Geometry: final body of the model. Coordinates: model frame, mm. A direction names the side the tool comes from. Give positions to 0.01 mm unless a question says otherwise; leave off trailing zeros. Loops run counter-clockwise (first coordinate to the right, second up) from the corner with the lowest first, then second, coordinate; pieces in that order, holes last. Notation, with made-up numbers: (79.25, 9) -> (99.25, 9) arc R13 cw to (99.25, 26) -> close; hole circle Ø3 at (12, 8.5). An arc over 180 degrees is marked (long way). Answer in a Markdown table with one row per item. Add a question column.
1) Section query B-B (x = -6). Return the cut outline in (y, z) (3 decimals).
2) Section query C-C (z = 23). Return the cut outline in (x, y) (3 decimals).
3) Access query for faces 4 (the cylindrical face through (-8.136, -0.954, 112.816)), 5 (the flat face through (8, 0, 90.998)). Directions: +Z, -Z, +X, -X, +Y, -Y. A direction counts if a zero-diameter tool reaches every point of the face in a straight line with its end or side. Return the directions, or none.
4) First-contact query: P1, Ø2, axis at x = -30.5, y = -1, coming from the -Z side; P2, Ø1.9, axis at x = 7, y = -1.5, coming from the +Z side; P3, Ø1, axis at y = 1.5, z = 59, coming from the -X side. Flat tips, straight axial feed; report the tip coordinate or a pass-through.
5) Section query A-A (y = 0). Return the cut outline in (x, z).
6) Line query: line 1 (Z direction, x = -16, y = 1.75); line 2 (X direction, y = -0.25, z = 57); line 3 (Z direction, x = -1, y = 1). Output: solid intervals per line, ascending. Write a range as from..to.
7) Draft query along X for faces 1 (the flat face through (8, 0, -90.998)), 2 (the cylindrical face through (-8.136, -0.954, -112.816)), 3 (the cylindrical face through (-31.02, -2.15, -98.66)). Return one class per face: +X half, -X half, draft (parallel to the pull), parting line (faces both ways), or undercut.
```python
from build123d import *

# Parameters (mm, degrees)
SKETCH3_R = 3.175


with BuildPart() as part:
    # Sweep1: sweep along a path in Sketch2
    with BuildLine(Plane(origin=(0, 0, 0), x_dir=(1, 0, 0), z_dir=(0, 1, 0))) as sweep1_path:
        Line((-42.005520706, 0), (-42.005520706, 74.510370248))
        ThreePointArc((-42.005520706, 74.510370248), (-41.43579821, 78.271535981), (-39.777746269, 81.695249631))
        Line((-39.777746269, 81.695249631), (-18.645117879, 112.496831598))
        ThreePointArc((-18.645117879, 112.496831598), (-15.912495952, 114.928072333), (-12.361782541, 115.805903968))
        Line((-12.361782541, 115.805903968), (-4.027166859, 115.805903968))
        ThreePointArc((-4.027166859, 115.805903968), (4.766000348, 112.163654854), (8.408249461, 103.370487647))
        Line((8.408249461, 103.370487647), (8.408249461, 90.998440491))
    # Sketch3 → Sweep1 (sweep)
    with BuildSketch(Plane.XY):
        with Locations((-42.04385452, 0)):
            Circle(SKETCH3_R)
    sweep1 = sweep(path=sweep1_path.line)

    # Mirror2: Sweep1 across plane
    add(sweep1.mirror(Plane(origin=(-42.04385452, 0, 0), x_dir=(1, 0, 0), z_dir=(0, 0, 1))))


solid = part.part
```
Evaluation:
| question | item | result |
|---|---|---|
| 1 | outline | circle Ø6.35 at (0, -115.844); circle Ø6.35 at (0, 115.844) |
| 2 | outline | circle Ø6.35 at (-42.044, 0) |
| 3 | face 4 | none |
| 3 | face 5 | +X, +Y, -Y |
| 4 | P1 | z = -102.15 |
| 4 | P2 | z = 115.01 |
| 4 | P3 | x = -45.06 |
| 5 | outline | (-45.22, -74.51) arc R15.91 ccw to (-42.43, -83.51) -> (-21.29, -114.31) arc R10.83 ccw to (-12.36, -119.02) -> (-4.03, -119.02) arc R15.65 ccw to (11.62, -103.37) -> (11.62, -91) -> (5.27, -91) -> (5.27, -103.37) arc R9.3 cw to (-4.03, -112.67) -> (-12.36, -112.67) arc R4.48 cw to (-16.06, -110.72) -> (-37.19, -79.92) arc R9.56 cw to (-38.87, -74.51) -> (-38.87, 74.51) arc R9.56 cw to (-37.19, 79.92) -> (-16.06, 110.72) arc R4.48 cw to (-12.36, 112.67) -> (-4.03, 112.67) arc R9.3 cw to (5.27, 103.37) -> (5.27, 91) -> (11.62, 91) -> (11.62, 103.37) arc R15.65 ccw to (-4.03, 119.02) -> (-12.36, 119.02) arc R10.83 ccw to (-21.29, 114.31) -> (-42.43, 83.51) arc R15.91 ccw to (-45.22, 74.51) -> close |
| 6 | line 1 | -117.83..-111.63, 111.63..117.83 |
| 6 | line 2 | -45.21..-38.88 |
| 6 | line 3 | -118.56..-112.33, 112.33..118.56 |
| 7 | face 1 | draft |
| 7 | face 2 | undercut |
| 7 | face 3 | undercut |
